Read the model definition and answer for the solid it produces. Units are mm, in the model's axes. Coordinates: 2 decimals unless noted, no trailing zeros. Order: outer loops, then holes, each group sorted by start corner. A loop starts at its lowest first (then second) coordinate and runs counter-clockwise, first axis right, second up. Notation, with made-up numbers: M 33,41 L 43,41 A34 cw 43,77 Z; hole C 56.25,18 d10. An arc over 180 degrees is marked long. Use a Markdown table: item, result. Add a question column.
1) Find section D-D on z = 81.5. Write down the section's boundary in (x, y), plus the area to 3 significant figures.
2) Find section B-B on y = 1.2. Write down the section's boundary in (x, z), plus the area to 3 significant figures.
3) This flat-tipped pin is pushed along its axis until it touches: pin 1 Ø16.5 at (x, z) = (5.5, 45) entering from +Y. Where does it stop, or does it pass through?
4) Find section C-C on z = 11.5. Write down the section's boundary in (x, y), plus the area to 3 significant figures.
5) Find the intervals of material crossed by probe 1 along Z at (x, y) = (-12.35, -0.1); probe 2 along X at (y, z) = (0.5, 31); probe 3 along Y at (x, z) = (20.5, 18), in increasing order. Write a range as [from, to].
6) Find section A-A on x = 12.35. Write down the section's boundary in (y, z), plus the area to 3 significant figures.
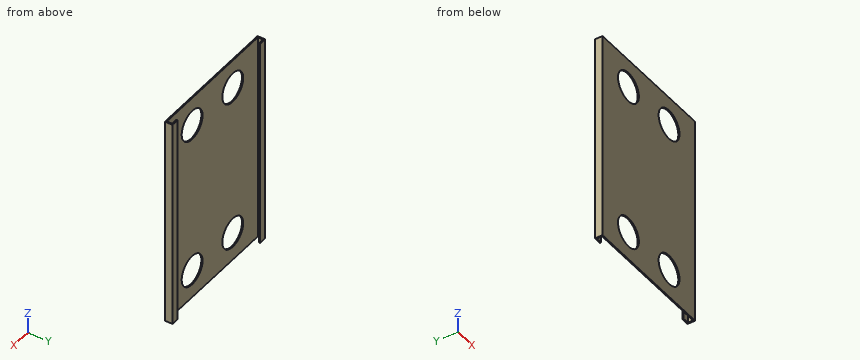
from build123d import *

# Parameters (mm, degrees)
EXTRUDE_THIN3_DEPTH     = 89.154
CUT_EXTRUDE1_DEPTH      = 94.54354816
CUT_EXTRUDE1_DEPTH_BACK = 94.54354816
SKETCH8_R               = 6.35


with BuildPart() as part:
    # Sketch6 → Extrude-Thin3 (new body)
    with BuildSketch(Plane.XY):
        Polygon((25.0952, 2.1336), (27.6352, 2.1336), (27.6352, 0), (-27.6352, 0), (-27.6352, 2.1336), (-25.0952, 2.1336), (-25.0952, 2.6416), (-28.1432, 2.6416), (-28.1432, -0.508), (28.1432, -0.508), (28.1432, 2.6416), (25.0952, 2.6416), align=None)
    extrude(amount=EXTRUDE_THIN3_DEPTH)

    # Sketch8 → Cut-Extrude1 (cut, two sides: drawn at the far end of the back side and taken through both)
    with BuildSketch(Plane.XZ.offset(0.508).offset(-CUT_EXTRUDE1_DEPTH_BACK)):
        with Locations(Location((12.35, 77.077, 0), (0, 0, 270))):
            Circle(SKETCH8_R)
        with Locations(Location((-12.35, 77.077, 0), (0, 0, 270))):
            Circle(SKETCH8_R)
        with Locations(Location((-12.35, 12.077, 0), (0, 0, 270))):
            Circle(SKETCH8_R)
        with Locations(Location((12.35, 12.077, 0), (0, 0, 270))):
            Circle(SKETCH8_R)
    extrude(amount=CUT_EXTRUDE1_DEPTH + CUT_EXTRUDE1_DEPTH_BACK, mode=Mode.SUBTRACT)


solid = part.part
Check result:
| question | item | result |
|---|---|---|
| 1 | outline | M -28.14,-0.51 L -16.91,-0.51 L -16.91,0 L -27.64,0 L -27.64,2.13 L -25.1,2.13 L -25.1,2.64 L -28.14,2.64 Z; M -7.79,-0.51 L 7.79,-0.51 L 7.79,0 L -7.79,0 Z; M 16.91,-0.51 L 28.14,-0.51 L 28.14,2.64 L 25.1,2.64 L 25.1,2.13 L 27.64,2.13 L 27.64,0 L 16.91,0 Z |
| 1 | area | 24.6 mm2 |
| 2 | outline | M -28.14,0 L -27.64,0 L -27.64,89.15 L -28.14,89.15 Z; M 27.64,0 L 28.14,0 L 28.14,89.15 L 27.64,89.15 Z |
| 2 | area | 90.6 mm2 |
| 3 | pin 1 | stops at y = 0 |
| 4 | outline | M -28.14,-0.51 L -18.67,-0.51 L -18.67,0 L -27.64,0 L -27.64,2.13 L -25.1,2.13 L -25.1,2.64 L -28.14,2.64 Z; M -6.03,-0.51 L 6.03,-0.51 L 6.03,0 L -6.03,0 Z; M 18.67,-0.51 L 28.14,-0.51 L 28.14,2.64 L 25.1,2.64 L 25.1,2.13 L 27.64,2.13 L 27.64,0 L 18.67,0 Z |
| 4 | area | 21.0 mm2 |
| 5 | probe 1 | z = [0, 5.73], [18.43, 70.73], [83.43, 89.15] |
| 5 | probe 2 | x = [-28.14, -27.64], [27.64, 28.14] |
| 5 | probe 3 | y = [-0.51, 0] |
| 6 | outline | M -0.51,0 L 0,0 L 0,5.73 L -0.51,5.73 Z; M -0.51,18.43 L 0,18.43 L 0,70.73 L -0.51,70.73 Z; M -0.51,83.43 L 0,83.43 L 0,89.15 L -0.51,89.15 Z |
| 6 | area | 32.4 mm2 |
